```python
from build123d import *

# Parameters (mm, degrees)
BOSS_EXTRUDE1_DEPTH = 6
HOLE1_D             = 4
HOLE1_DEPTH         = 3
HOLE1_CBORE_D       = 5
HOLE1_CBORE_DEPTH   = 0.8
HOLE1_TIP           = 1.201721238
HOLE2_D             = 4
HOLE2_DEPTH         = 18
HOLE2_CBORE_D       = 5
HOLE2_CBORE_DEPTH   = 0.8
HOLE2_TIP           = 1.201721238
CUT_EXTRUDE1_START  = -0.8
CUT_EXTRUDE1_DEPTH  = 0.8
CUT_EXTRUDE2_DEPTH  = 0.8
CUT_EXTRUDE3_START  = -0.8
SKETCH8_R           = 2.5
CUT_EXTRUDE3_DEPTH  = 0.8
CHAMFER1_START      = -12
CHAMFER1_OUTLINE_W  = 5
CHAMFER1_OUTLINE_H  = 6
CHAMFER1_DEPTH      = 2.524769132
FILLET1_R           = 3


with BuildPart() as part:
    # Sketch1 → Boss-Extrude1 (new body)
    with BuildSketch(Plane.XY):
        Polygon((0, 0), (-15, 0), (-15, 18), (-12, 18), (-12, 3), (0, 3), align=None)
    extrude(amount=BOSS_EXTRUDE1_DEPTH)

    # Hole1
    with Locations(Plane(origin=(-12, 0, 0), x_dir=(0, 0, -1), z_dir=(1, 0, 0))):
        with Locations((-3, 9), (-3, 15)):
            CounterBoreHole(HOLE1_D / 2, HOLE1_CBORE_D / 2, HOLE1_CBORE_DEPTH, depth=HOLE1_DEPTH)
            with Locations((0, 0, -(HOLE1_DEPTH + HOLE1_TIP / 2))):  # 118° drill point
                Cone(0, HOLE1_D / 2, HOLE1_TIP, mode=Mode.SUBTRACT)

    # Hole2
    with Locations(Plane(origin=(0, 0, 0), x_dir=(-1, 0, 0), z_dir=(0, -1, 0))):
        with Locations((9, -3), (3, -3)):
            CounterBoreHole(HOLE2_D / 2, HOLE2_CBORE_D / 2, HOLE2_CBORE_DEPTH, depth=HOLE2_DEPTH)
            with Locations((0, 0, -(HOLE2_DEPTH + HOLE2_TIP / 2))):  # 118° drill point
                Cone(0, HOLE2_D / 2, HOLE2_TIP, mode=Mode.SUBTRACT)

    # Sketch6 → Cut-Extrude1 (cut)
    with BuildSketch(Plane(origin=(0, 3, 0), x_dir=(1, 0, 0), z_dir=(0, 1, 0)).offset(CUT_EXTRUDE1_START)):
        with BuildLine():
            Line((-9, -0.5), (0, -0.5))
            Line((0, -0.5), (0, -5.5))
            Line((0, -5.5), (-9, -5.5))
            ThreePointArc((-9, -5.5), (-11.5, -3), (-9, -0.5))
        make_face()
    extrude(amount=CUT_EXTRUDE1_DEPTH, mode=Mode.SUBTRACT)

    # Sketch7 → Cut-Extrude2 (cut)
    with BuildSketch(Plane.XZ):
        with BuildLine():
            Line((-15, 5.35), (-15, 0.65))
            ThreePointArc((-15, 0.65), (-12.65, 3), (-15, 5.35))
        make_face()
    extrude(amount=-CUT_EXTRUDE2_DEPTH, mode=Mode.SUBTRACT)

    # Sketch8 → Cut-Extrude3 (cut)
    with BuildSketch(Plane.ZY.offset(15).offset(CUT_EXTRUDE3_START)):
        with Locations(Location((3, 9, 0), (0, 0, 180))):
            Circle(SKETCH8_R)
        with Locations(Location((3, 15, 0), (0, 0, 180))):
            Circle(SKETCH8_R)
        with BuildLine():
            Line((0.5, 3), (0.5, 0))
            Line((0.5, 0), (5.5, 0))
            Line((5.5, 0), (5.5, 3))
            ThreePointArc((5.5, 3), (3, 5.5), (0.5, 3))
        make_face()
    extrude(amount=CUT_EXTRUDE3_DEPTH, mode=Mode.SUBTRACT)

    # Chamfer1: read off the stored shape, not the designer's step
    # Chamfer1 outline → Chamfer1 (cut)
    with BuildSketch(Plane(origin=(0, 0, 0), x_dir=(0.707106781186546, -0.707106781186549, 0), z_dir=(0.707106781186549, 0.707106781186546, 0)).offset(CHAMFER1_START)):
        with Locations((-10.5, -3)):
            Rectangle(CHAMFER1_OUTLINE_W, CHAMFER1_OUTLINE_H)
    extrude(amount=CHAMFER1_DEPTH, mode=Mode.SUBTRACT)

    # Fillet1
    fillet1_edges = [part.edges().sort_by_distance(p)[0] for p in [
        (0, 1.5, 6),
        (-13.5, 18, 6),
    ]]
    fillet(fillet1_edges, radius=FILLET1_R)

    # Mirror1: part across plane


with BuildPart() as part_1:
    add(part.part)
    add(part.part.mirror(Plane.XY))


solid = part_1.part
```
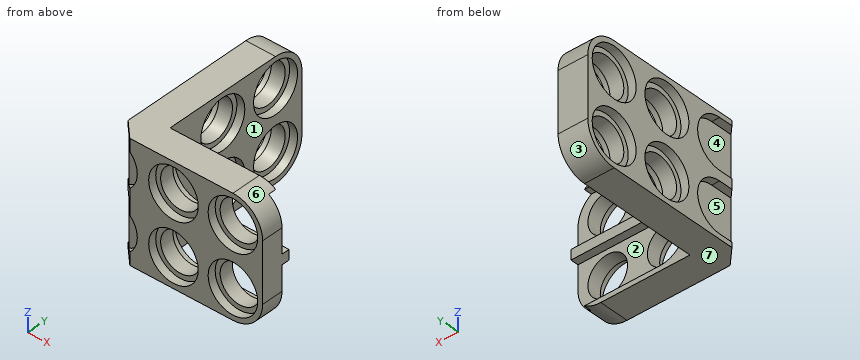
Source: CAD feature listing. Evaluate the final solid. Frame: model axes, mm. Face numbers are marked on the shaded views. A direction names the side the tool comes from. Round coordinates to 2 decimals unless told otherwise and drop trailing zeros. Write each loop counter-clockwise with the first axis right and the second up, starting at its lowest first coordinate (ties: lowest second). Pieces come first, ordered by that corner, then holes. Notation, with made-up numbers: M 37.25,-20 L 89.25,-20 A31 ccw 89.25,12 Z; hole C 19.5,14 d3. An arc over 180 degrees is marked long. Use CSV: the item, a comma, the result in double quotes. Start each with the question number.
Q1. Cut plane C-C on y = 2.5. Output: boundary loops of the cut face in (x, z), plus the area to 3 significant figures.
Q2. First-contact query: P1, Ø6, axis at y = 5, z = -2, coming from the +X side; P2, Ø3, axis at x = -9, z = 3, coming from the -Y side; P3, Ø0.8, axis at x = -13.5, z = -3, coming from the -Y side; P4, Ø1, axis at y = 10.5, z = 1.5, coming from the +X side. Flat tips, straight axial feed; report the tip coordinate or a pass-through.
Q3. Access query for the marked faces 1, 2 and 3. Directions: +Z, -Z, +X, -X, +Y, -Y. A direction counts if a zero-diameter tool reaches every point of the face in a straight line with its end or side. Return the directions, or none.
Q4. Cut plane D-D on z = 4.5. Count the separate pieces of the cut face and the enclosed holes in it, plus the area to 3 significant figures.
Q5. Pull-direction query (Z, two-part tool) for the marked faces 4, 5, 6 and 7; classes: +Z half, -Z half, draft (parallel to the pull), parting line (faces both ways), or undercut.
Q6. Cut plane A-A on y = 9. Output: boundary loops of the cut face in (x, z), plus the area to 3 significant figures.
Q7. Line query: line 1 (Z direction, x = -9, y = 0.6); line 2 (Y direction, x = -13.5, z = -3); line 3 (Y direction, x = -12.3, z = -3). Output: solid intervals per line, ascending. Write a range as from..to.
Q8. Cut plane B-B on x = -7.5. Output: boundary loops of the cut face in (y, z), plus the area to 3 significant figures.
Results found:
1,outline,"M -15,-6 L -3,-6 A3 ccw -1.34,-5.5 L -9,-5.5 A2.5 cw -9,-0.5 L 0,-0.5 L 0,0.5 L -9,0.5 A2.5 cw -9,5.5 L -1.34,5.5 A3 ccw -3,6 L -15,6 L -15,5.5 L -14.2,5.5 L -14.2,0.5 L -15,0.5 L -15,-0.5 L -14.2,-0.5 L -14.2,-5.5 L -15,-5.5 Z"
1,area,"60.5 mm^2"
2,P1,"x = 0"
2,P2,"through"
2,P3,"y = 0.8"
2,P4,"x = -12"
3,face 1,"+Z, -Z, +X, +Y"
3,face 2,"+X, +Y"
3,face 3,"-Z, +X, -X, +Y"
4,separate pieces,"5"
4,enclosed holes,"0"
4,area,"40.3 mm^2"
5,face 4,"undercut"
5,face 5,"undercut"
5,face 6,"+Z half"
5,face 7,"-Z half"
6,outline,"M -15,-6 L -12,-6 L -12,-5.5 L -12.8,-5.5 L -12.8,-5 L -14.2,-5 L -14.2,-5.5 L -15,-5.5 Z; M -15,-0.5 L -14.2,-0.5 L -14.2,-1 L -12.8,-1 L -12.8,-0.5 L -12,-0.5 L -12,0.5 L -12.8,0.5 L -12.8,1 L -14.2,1 L -14.2,0.5 L -15,0.5 Z; M -15,5.5 L -14.2,5.5 L -14.2,5 L -12.8,5 L -12.8,5.5 L -12,5.5 L -12,6 L -15,6 Z"
6,area,"8.80 mm^2"
7,line 1,"-6..-5.5, -0.5..0.5, 5.5..6"
7,line 2,"0.8..7, 11..13, 17..18"
7,line 3,"0..6.5, 11.5..12.5, 17.5..18"
8,outline,"M 0,-6 L 3,-6 L 3,-5.5 L 2.2,-5.5 L 2.2,-4.32 L 0.8,-4.32 L 0.8,-5 L 0,-5 Z; M 0,-1 L 0.8,-1 L 0.8,-1.68 L 2.2,-1.68 L 2.2,-0.5 L 3,-0.5 L 3,0.5 L 2.2,0.5 L 2.2,1.68 L 0.8,1.68 L 0.8,1 L 0,1 Z; M 0,5 L 0.8,5 L 0.8,4.32 L 2.2,4.32 L 2.2,5.5 L 3,5.5 L 3,6 L 0,6 Z"
8,area,"14.2 mm^2"
